```python
from build123d import *

# Parameters (mm, degrees)
F0_R      = 100
F1_DEPTH  = 28
F2_R      = 65
F2_R_2    = 37.5
F3_DEPTH  = 15
F5_DEPTH  = 10
F6_R      = 6
F7_DEPTH  = 2
F3_FACE_R = 37.5
F8_DEPTH  = 50
F9_SIZE   = 5


with BuildPart() as f1:
    # F0 (on Top) → F1 (new body)
    with BuildSketch(Plane.XY):
        Circle(F0_R)
    extrude(amount=F1_DEPTH)

    # F2 (on face) → F3 (join)
    with BuildSketch(Plane(origin=(0, 0, 0), x_dir=(1, 0, 0), z_dir=(0, 0, -1))):
        Circle(F2_R)
        Circle(F2_R_2, mode=Mode.SUBTRACT)
    extrude(amount=F3_DEPTH)

    # F4 (on face) → F5 (join)
    with BuildSketch(Plane(origin=(0, 0, -15), x_dir=(1, 0, 0), z_dir=(0, 0, -1))):
        with BuildLine():
            ThreePointArc((-65, 0), (-64.695978, -6.27937), (-63.786754, -12.5))
            Line((-63.786754, -12.5), (-40, -12.5))
            Line((-40, -12.5), (-40, 12.5))
            Line((-40, 12.5), (-63.786754, 12.5))
            ThreePointArc((-63.786754, 12.5), (-64.695978, 6.27937), (-65, 0))
        make_face()
        with BuildLine():
            Line((40, -12.5), (63.786754, -12.5))
            ThreePointArc((63.786754, -12.5), (64.695978, -6.27937), (65, 0))
            ThreePointArc((65, 0), (64.695978, 6.27937), (63.786754, 12.5))
            Line((63.786754, 12.5), (40, 12.5))
            Line((40, 12.5), (40, -12.5))
        make_face()
        with BuildLine():
            ThreePointArc((63.786754, 12.5), (64.695978, 6.27937), (65, 0))
            Line((65, 0), (65, 12.5))
            Line((65, 12.5), (63.786754, 12.5))
        make_face()
        with BuildLine():
            Line((63.786754, -12.5), (65, -12.5))
            Line((65, -12.5), (65, 0))
            ThreePointArc((65, 0), (64.695978, -6.27937), (63.786754, -12.5))
        make_face()
        with BuildLine():
            Line((-65, 12.5), (-65, 0))
            ThreePointArc((-65, 0), (-64.695978, 6.27937), (-63.786754, 12.5))
            Line((-63.786754, 12.5), (-65, 12.5))
        make_face()
        with BuildLine():
            Line((-65, -12.5), (-63.786754, -12.5))
            ThreePointArc((-63.786754, -12.5), (-64.695978, -6.27937), (-65, 0))
            Line((-65, 0), (-65, -12.5))
        make_face()
    extrude(amount=F5_DEPTH)

    # F6 (on face) → F7 (cut)
    with BuildSketch(Plane(origin=(0, 0, -25), x_dir=(1, 0, 0), z_dir=(0, 0, -1))):
        with Locations((52.5, 0)):
            Circle(F6_R)
        with Locations((-52.5, 0)):
            Circle(F6_R)
    extrude(amount=-F7_DEPTH, mode=Mode.SUBTRACT)

    # F3_face (on face) → F8 (cut)
    with BuildSketch(Plane(origin=(0, 0, -15), x_dir=(1, 0, 0), z_dir=(0, 0, -1))):
        Circle(F3_FACE_R)
    extrude(amount=-F8_DEPTH, mode=Mode.SUBTRACT)

    # F9
    f9_edges = [f1.edges().sort_by_distance(p)[0] for p in [
        (-100, 0, 0),
    ]]
    chamfer(f9_edges, length=F9_SIZE)


solid = f1.part
```
CAD build for the part. Positions are in the model's coordinates, mm. A direction names the side the tool comes from. Coordinates: 2 decimals unless noted, no trailing zeros. Order: outer loops, then holes, each group sorted by start corner. A loop starts at its lowest first (then second) coordinate and runs counter-clockwise, first axis right, second up.
(1) Which spindle directions (+Z, -Z, +X, -X, +Y, -Y) get a long thin tool onto all of the face, cutting with end or side? Do faces 5 (the face through (-53, 12.5, -20)), 6 (the face through (-65, 0, -20)), 7 (the face through (52, 0, -23)), 8 (the face through (40, 0, -20)), 9 (the face through (-52, -12.5, -20)). Say none if no direction does.
Solution:
face 5: -Z, +X, -X, +Y
face 6: -Z, -X, +Y, -Y
face 7: -Z
face 8: -Z, +Y, -Y
face 9: -Z, +X, -X, -Y
(2) Drill centre lines: L1, parallel to X at y = 0, z = -23.95; L2, parallel to Y at x = 52.5, z = -24.4; L3, parallel to Y at x = 0, z = -9. Where is each one in solid material? Low to high.
Solution:
L1: x = -65 to -58.5, -46.5 to -40, 40 to 46.5, 58.5 to 65
L2: y = -12.5 to -6, 6 to 12.5
L3: y = -65 to -37.5, 37.5 to 65
(3) Saw through at B-B, the plane z = -10.5. Write the cut outline in (x, y), and give its area (3 significant figures).
Solution:
outline: circle Ø130 at (0, 0); hole circle Ø75 at (0, 0)
area: 8,860 mm2
(4) Saw through at C-C, the plane z = 21. Write the cut outline in (x, y).
Solution:
outline: circle Ø200 at (0, 0); hole circle Ø75 at (0, 0)
(5) Mould opens along X. For faces 1 (the face through (-58.494, -0.264, -24.014)), 2 (the face through (65, 0, -20)), 3 (the face through (-40, 0, -20)), 4 (the face through (-58, -3, -25)) say: released by +X, released by -X, zero draft, split by the parting line, or undercut.
Solution:
face 1: undercut
face 2: released by +X
face 3: undercut
face 4: zero draft
(6) Saw through at A-A, the plane x = 0. Write the cut outline in (y, z), and give its area (3 significant figures).
Solution:
outline: (-100, 5) - (-95, 0) - (-65, 0) - (-65, -15) - (-37.5, -15) - (-37.5, 28) - (-100, 28) - close; (37.5, -15) - (65, -15) - (65, 0) - (95, 0) - (100, 5) - (100, 28) - (37.5, 28) - close
area: 4,300 mm2
(7) Pin check, flat tips, straight feed: pin 1 Ø5 at (x, z) = (16, 14.5) entering from +Y; pin 2 Ø2 at (y, z) = (59, 15.5) entering from -X; pin 3 Ø1.5 at (x, z) = (8.5, -3) entering from +Y. Stop position of each tip, or through.
Solution:
pin 1: stops at y = 99.08
pin 2: stops at x = -81.46
pin 3: stops at y = 64.54
